Input: dimensioned drawing with shaded views. Units: mm. Origin: part minimum x, y, z. A direction names the side the tool comes from. Round coordinates to 2 decimals unless told otherwise and drop trailing zeros. Order: outer loops, then holes, each group sorted by start corner. A loop starts at its lowest first (then second) coordinate and runs counter-clockwise, first axis right, second up.
Item 1: Line query: L1, parallel to Y at x = 6.5, z = 2 (1 decimal); L2, parallel to Z at x = 7.5, y = 13.5; L3, parallel to X at y = 6.5, z = 3 (1 decimal). Output: solid intervals per line, ascending.
Item 2: Cut plane C-C on z = 7. Output: boundary loops of the cut face in (x, y).
Item 3: Reachability of the marked faces 1 and 2 from +Z, -Z, +X, -X, +Y, -Y: full face, straight path, thin tool, end or side. Return the list, or none.
Item 4: First-contact query: pin 1 (3 mm diameter, centred on y = 9, z = 7.5, fed in from +X); pin 2 (1.5 mm diameter, centred on y = 5.5, z = 18, fed in from +X); pin 3 (6 mm diameter, centred on x = 2.5, z = 27.5, fed in from -Y). Flat tips, straight axial feed; report the tip coordinate or a pass-through.
Item 5: Cut plane D-D on y = 2.5. Output: boundary loops of the cut face in (x, z).
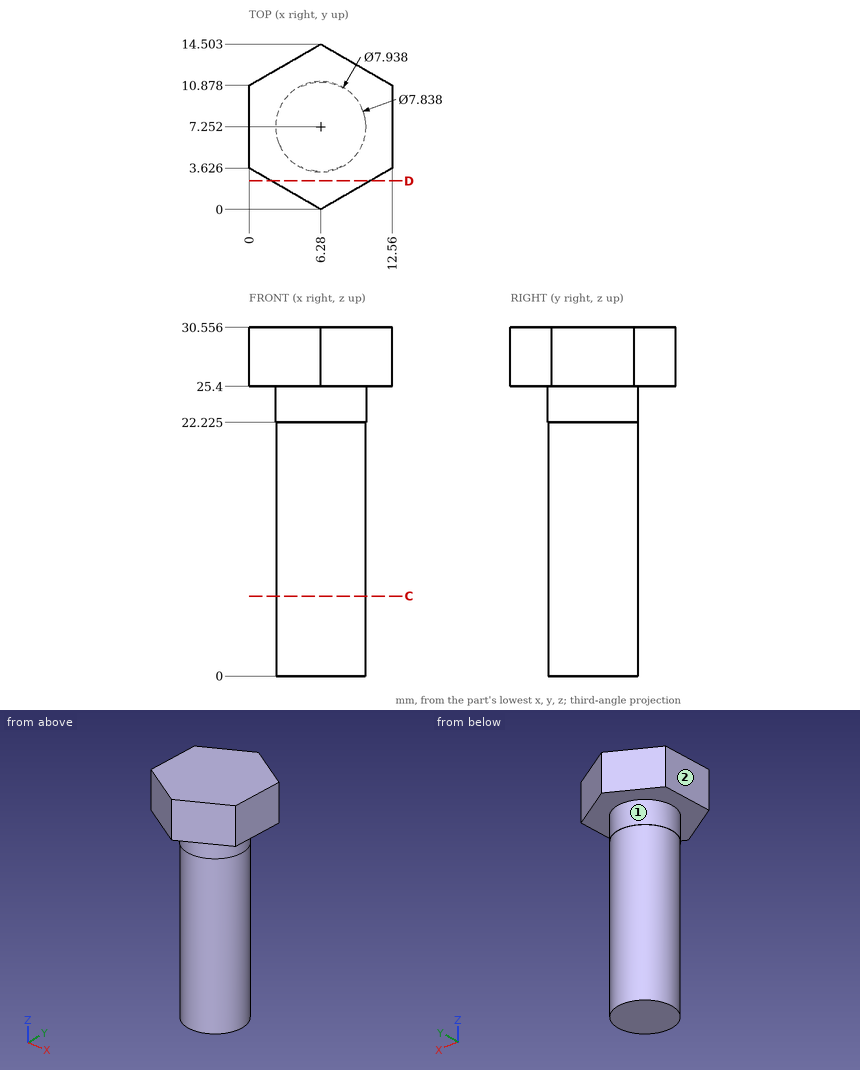
From the geometry:
1. L1: y = 3.3 to 11.2
1. L2: z = 25.4 to 30.56
1. L3: x = 2.4 to 10.1
2. outline: circle Ø7.84 at (6.28, 7.25)
3. face 1: -Z
3. face 2: +Z, -Z, -X, +Y, -Y
4. pin 1: stops at x = 10.19
4. pin 2: stops at x = 10.07
4. pin 3: stops at y = 0.45
5. outline: (1.95, 25.4) - (10.61, 25.4) - (10.61, 30.56) - (1.95, 30.56) - close
